```python
from build123d import *

# Parameters (mm, degrees)
SKETCH1_W           = 36.9
SKETCH1_H           = 32.9
SKETCH1_R           = 1.5
BOSS_EXTRUDE1_DEPTH = 2
BOSS_EXTRUDE2_DEPTH = 42
SKETCH5_W           = 2.5
SKETCH5_H           = 10
BOSS_EXTRUDE3_DEPTH = 10
FILLET1_R           = 1
CUT_EXTRUDE1_REACH  = 9
SKETCH3_R           = 1.15
SKETCH3_W           = 22
SKETCH3_H           = 12.25


with BuildPart() as part:
    # Sketch1 → Boss-Extrude1 (new body)
    with BuildSketch(Plane.XY):
        with Locations((18.45, 16.45)):
            Rectangle(SKETCH1_W, SKETCH1_H)
        with Locations((18.45, 16.45)):
            Circle(SKETCH1_R, mode=Mode.SUBTRACT)
    extrude(amount=BOSS_EXTRUDE1_DEPTH)

    # Sketch2 → Boss-Extrude2 (add)
    with BuildSketch(Plane.XY.offset(2)):
        Polygon((3.5, 0), (7, 0), (7, 30.4), (36.9, 30.4), (36.9, 32.9), (3.5, 32.9), align=None)
    extrude(amount=BOSS_EXTRUDE2_DEPTH)

    # Sketch5 → Boss-Extrude3 (add)
    with BuildSketch(Plane.XY.offset(2)):
        with Locations((35.65, 15)):
            Rectangle(SKETCH5_W, SKETCH5_H)
    extrude(amount=BOSS_EXTRUDE3_DEPTH)

    # Fillet1
    fillet1_edges = [part.edges().sort_by_distance(p)[0] for p in [
        (3.5, 16.45, 2),
        (7, 15.2, 2),
        (21.95, 30.4, 2),
        (7, 30.4, 23),
        (36.9, 30.4, 23),
        (3.5, 16.45, 44),
        (5.25, 0, 44),
        (7, 15.2, 44),
        (21.95, 30.4, 44),
        (36.9, 31.65, 44),
        (20.2, 32.9, 44),
        (36.9, 25.2, 2),
        (36.9, 10, 7),
        (35.65, 20, 2),
        (36.9, 20, 7),
        (34.4, 15, 2),
        (34.4, 20, 7),
        (35.65, 10, 2),
        (34.4, 10, 7),
        (36.9, 15, 12),
        (35.65, 20, 12),
        (34.4, 15, 12),
        (35.65, 10, 12),
        (36.9, 5, 2),
        (36.9, 0, 1),
        (0, 0, 1),
        (0, 32.9, 1),
        (36.9, 32.9, 22),
    ]]
    fillet(fillet1_edges, radius=FILLET1_R)

    # Sketch3 → Cut-Extrude1 (cut, up to next)
    with BuildSketch(Plane(origin=(7, 0, 0), x_dir=(0, 0, -1), z_dir=(1, 0, 0)), mode=Mode.PRIVATE) as cut_extrude1_sk1:
        with Locations((-39.215, 27.4)):
            Circle(SKETCH3_R)
    cut_extrude1_tool1 = extrude(cut_extrude1_sk1.sketch, amount=-CUT_EXTRUDE1_REACH, mode=Mode.PRIVATE) & part.part
    add(cut_extrude1_tool1.solids().sort_by_distance((7, 27.4, 39.215))[0], mode=Mode.SUBTRACT)
    # Sketch3 → Cut-Extrude1 (cut, up to next)
    with BuildSketch(Plane(origin=(7, 0, 0), x_dir=(0, 0, -1), z_dir=(1, 0, 0)), mode=Mode.PRIVATE) as cut_extrude1_sk2:
        with Locations((-17.685, 27.4)):
            Circle(SKETCH3_R)
    cut_extrude1_tool2 = extrude(cut_extrude1_sk2.sketch, amount=-CUT_EXTRUDE1_REACH, mode=Mode.PRIVATE) & part.part
    add(cut_extrude1_tool2.solids().sort_by_distance((7, 27.4, 17.685))[0], mode=Mode.SUBTRACT)
    # Sketch3 → Cut-Extrude1 (cut, up to next)
    with BuildSketch(Plane(origin=(7, 0, 0), x_dir=(0, 0, -1), z_dir=(1, 0, 0)), mode=Mode.PRIVATE) as cut_extrude1_sk3:
        with Locations((-39.215, 14.9)):
            Circle(SKETCH3_R)
    cut_extrude1_tool3 = extrude(cut_extrude1_sk3.sketch, amount=-CUT_EXTRUDE1_REACH, mode=Mode.PRIVATE) & part.part
    add(cut_extrude1_tool3.solids().sort_by_distance((7, 14.9, 39.215))[0], mode=Mode.SUBTRACT)
    # Sketch3 → Cut-Extrude1 (cut, up to next)
    with BuildSketch(Plane(origin=(7, 0, 0), x_dir=(0, 0, -1), z_dir=(1, 0, 0)), mode=Mode.PRIVATE) as cut_extrude1_sk4:
        with Locations((-17.685, 14.9)):
            Circle(SKETCH3_R)
    cut_extrude1_tool4 = extrude(cut_extrude1_sk4.sketch, amount=-CUT_EXTRUDE1_REACH, mode=Mode.PRIVATE) & part.part
    add(cut_extrude1_tool4.solids().sort_by_distance((7, 14.9, 17.685))[0], mode=Mode.SUBTRACT)
    # Sketch3 → Cut-Extrude1 (cut, up to next)
    with BuildSketch(Plane(origin=(7, 0, 0), x_dir=(0, 0, -1), z_dir=(1, 0, 0)), mode=Mode.PRIVATE) as cut_extrude1_sk5:
        with Locations((-28.45, 6.125)):
            Rectangle(SKETCH3_W, SKETCH3_H)
    cut_extrude1_tool5 = extrude(cut_extrude1_sk5.sketch, amount=-CUT_EXTRUDE1_REACH, mode=Mode.PRIVATE) & part.part
    add(cut_extrude1_tool5.solids().sort_by_distance((7, 6.125, 28.45))[0], mode=Mode.SUBTRACT)


solid = part.part
```
CAD build for the part. Positions are in the model's coordinates, mm. A direction names the side the tool comes from. Coordinates: 2 decimals unless noted, no trailing zeros. Write each loop counter-clockwise with the first axis right and the second up, starting at its lowest first coordinate (ties: lowest second). Pieces come first, ordered by that corner, then holes.
(1) Cut at B-B, the plane x = 18.45. List the corners of the cut face in (y, z).
(2) Cut at D-D, the plane x = 11.5. List the corners of the cut face in (y, z).
(3) Flat gauge pins, fed straight in: pin 1 (10 mm diameter, centred on y = 24.5, z = 30, fed in from -X); pin 2 (1.2 mm diameter, centred on x = 1.5, y = 10.5, fed in from +Z); pin 3 (4 mm diameter, centred on x = 9.5, z = 23.5, fed in from -Y). Where does each tip first touch, or does it go through?
(4) 3-axis set-ups, long thin cutter, end or side, ignore diameter. For faces 1 (the face through (36.615, 15.056, 11.699)), 2 (the face through (1, 17, 2)), 3 (the face through (5, 12.25, 29)), 4 (the face through (36.615, 19.699, 7.056)): which of +Z, -Z, +X, -X, +Y, -Y reach the whole face in a straight line?
(5) Drill centre lines: probe 1 along X at (y, z) = (12.5, 7); probe 2 along Z at (x, y) = (5, 14); probe 3 along Y at (x, z) = (18.45, 1). Where is each one in solid material? Low to high.
(6) Two-plate mould, pull along Y, no slides. Class faces 5 (the face through (5, 6, 17.45)), 6 (the face through (36.615, 30.701, 23.28)), 7 (the face through (36.599, 0.285, 0.792)): +Y half, -Y half, draft (parallel to the pull), parting line (faces both ways), or undercut.
(7) Cut at C-C, the plane z = 41. List the corners of the cut face in (x, y), and give its area (3 significant figures).
(8) Cut at A-A, the plane y = 27.4. List the corners of the cut face in (x, z) (3 decimals).
Geometry says:
1. outline: (0, 0) - (14.95, 0) - (14.95, 2) - (0, 2) - close; (17.95, 0) - (32.9, 0) - (32.9, 43) arc R1 ccw to (31.9, 44) - (31.4, 44) arc R1 ccw to (30.4, 43) - (30.4, 3) arc R1 cw to (29.4, 2) - (17.95, 2) - close
2. outline: (0, 0) - (32.9, 0) - (32.9, 43) arc R1 ccw to (31.9, 44) - (31.4, 44) arc R1 ccw to (30.4, 43) - (30.4, 3) arc R1 cw to (29.4, 2) - (0, 2) - close
3. pin 1: stops at x = 3.5
3. pin 2: stops at z = 2
3. pin 3: stops at y = 30.27
4. face 1: +Z, +X, -Y
4. face 2: +Z, -X, +Y, -Y
4. face 3: +X, -X, -Y
4. face 4: +Z, +X
5. probe 1: x = 3.5 to 7, 34.4 to 36.9
5. probe 2: z = 0 to 16.97, 18.4 to 38.5, 39.93 to 44
5. probe 3: y = 0 to 14.95, 17.95 to 32.9
6. face 5: draft
6. face 6: undercut
6. face 7: -Y half
7. outline: (3.5, 0) - (7, 0) - (7, 29.4) arc R1 cw to (8, 30.4) - (35.9, 30.4) arc R1 ccw to (36.9, 31.4) - (36.9, 31.9) arc R1 ccw to (35.9, 32.9) - (3.5, 32.9) - close
7. area: 190 mm2
8. outline: (0, 0) - (36.9, 0) - (36.9, 1) arc R1 ccw to (35.9, 2) - (8, 2) arc R1 cw to (7, 3) - (7, 16.535) - (3.5, 16.535) - (3.5, 3) arc R1 cw to (2.5, 2) - (0, 2) - close; (3.5, 18.835) - (7, 18.835) - (7, 38.065) - (3.5, 38.065) - close; (3.5, 40.365) - (7, 40.365) - (7, 43) arc R1 ccw to (6, 44) - (4.5, 44) arc R1 ccw to (3.5, 43) - close
